Here's how the part is built. I have some questions about the finished solid (model axes, mm). Round coordinates to 2 decimals unless told otherwise and drop trailing zeros. Write each loop counter-clockwise with the first axis right and the second up, starting at its lowest first coordinate (ties: lowest second). Pieces come first, ordered by that corner, then holes. Notation, with made-up numbers: (44, 19) - (66, 19) arc R10 ccw to (66, 32) - close; hole circle Ø9 at (28.25, -27.75). An arc over 180 degrees is marked (long way). One line per question, with ' | ' between items. Start each with the question number.
(1) If I drill on L1, parallel to Y at x = -5, z = -1.25; L2, parallel to X at y = 5.75, z = -1.3; L3, parallel to Y at x = -3.75, z = -2.1, over which ranges is the centre line in solid material (lowest first)?
(2) Imagine slicing it at D-D (y = 7). Write out the boundary of the cut face in (x, z), plus the area to 3 significant figures.
(3) Imagine slicing it at A-A (y = 5). Write out the boundary of the cut face in (x, z).
(4) Imagine slicing it at C-C (z = -0.3). Write out the boundary of the cut face in (x, y).
(5) Imagine slicing it at B-B (x = -5). Write out the boundary of the cut face in (y, z), plus the area to 3 significant figures.
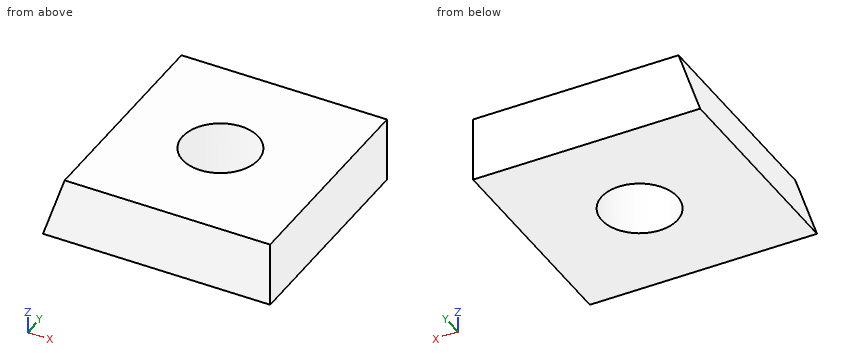
from build123d import *

# Parameters (mm, degrees)
BOSS_EXTRUDE1_DEPTH = 10
SKETCH2_R           = 1.75
CUT_EXTRUDE1_DEPTH  = 15.807092895


with BuildPart() as part:
    # Sketch1 → Boss-Extrude1 (new body)
    with BuildSketch(Plane(origin=(0, 0, 0), x_dir=(1, 0, 0), z_dir=(0, 1, 0))):
        Polygon((0, 0), (0, 3), (-10.5, 3), (-9.5, 0), align=None)
    extrude(amount=BOSS_EXTRUDE1_DEPTH)

    # Sketch2 → Cut-Extrude1 (cut, through all)
    with BuildSketch(Plane(origin=(0, 0, -3), x_dir=(-1, 0, 0), z_dir=(0, 0, -1))):
        with Locations((5, 5)):
            Circle(SKETCH2_R)
    extrude(amount=-CUT_EXTRUDE1_DEPTH, mode=Mode.SUBTRACT)


solid = part.part
Check sheet entries:
1) L1: 0 to 3.25, 6.75 to 10 | L2: -9.93 to -6.58, -3.42 to 0 | L3: 0 to 3.78, 6.22 to 10
2) outline: (-10.5, -3) - (0, -3) - (0, 0) - (-9.5, 0) - close | area: 30.0 mm^2
3) outline: (-10.5, -3) - (-6.75, -3) - (-6.75, 0) - (-9.5, 0) - close; (-3.25, -3) - (0, -3) - (0, 0) - (-3.25, 0) - close
4) outline: (-9.6, 0) - (0, 0) - (0, 10) - (-9.6, 10) - close; hole circle Ø3.5 at (-5, 5)
5) outline: (0, -3) - (3.25, -3) - (3.25, 0) - (0, 0) - close; (6.75, -3) - (10, -3) - (10, 0) - (6.75, 0) - close | area: 19.5 mm^2
